```python
from build123d import *

# Parameters (mm, degrees)
SKETCH_1_W           = 512
SKETCH_1_H           = 80
EXTRUDE_1_DEPTH      = 6
SKETCH_2_R           = 2.55
CUT_EXTRUDE_1_DEPTH  = 7
EXTRUDE_2_DEPTH      = 6
SKETCH_3_R           = 2.1
SKETCH_3_W           = 7
SKETCH_3_H           = 6
CUT_EXTRUDE_11_DEPTH = 7
EXTRUDE_21_DEPTH     = 6
SKETCH_31_R          = 2.1
SKETCH_31_W          = 7
SKETCH_31_H          = 6
CUT_EXTRUDE_12_DEPTH = 7
EXTRUDE_22_DEPTH     = 6
SKETCH_32_R          = 2.1
SKETCH_32_W          = 7
SKETCH_32_H          = 6
CUT_EXTRUDE_13_DEPTH = 7
EXTRUDE_23_DEPTH     = 6
SKETCH_33_R          = 2.1
SKETCH_33_W          = 7
SKETCH_33_H          = 6
CUT_EXTRUDE_14_DEPTH = 7
SKETCH_35_R          = 2.1
SKETCH_35_W          = 7
SKETCH_35_H          = 6
CUT_EXTRUDE_16_DEPTH = 7
EXTRUDE_25_DEPTH     = 6
SKETCH_36_R          = 2.1
SKETCH_36_W          = 7
SKETCH_36_H          = 6
CUT_EXTRUDE_17_DEPTH = 7
SKETCH_37_R          = 2.1
SKETCH_37_W          = 7
SKETCH_37_H          = 6
CUT_EXTRUDE_18_DEPTH = 7


with BuildPart() as part:
    # Эскиз1 → Бобышка-Вытянуть1 (new body)
    with BuildSketch(Plane.XY):
        with Locations((256, -204.461538462)):
            Rectangle(SKETCH_1_W, SKETCH_1_H)
    extrude(amount=EXTRUDE_1_DEPTH)

    # Эскиз2 → Вырез-Вытянуть1 (cut, through all)
    with BuildSketch(Plane.XY.offset(6)):
        with Locations((376, -234.461538462)):
            Circle(SKETCH_2_R)
        with Locations((376, -214.461538462)):
            Circle(SKETCH_2_R)
        with Locations((136, -234.461538462)):
            Circle(SKETCH_2_R)
        with Locations((136, -214.461538462)):
            Circle(SKETCH_2_R)
    extrude(amount=-CUT_EXTRUDE_1_DEPTH, mode=Mode.SUBTRACT)

    # Эскиз21 → Бобышка-Вытянуть2 (add)
    with BuildSketch(Plane(origin=(462, -227.461538462, 0), x_dir=(0, -1, 0), z_dir=(0, 0, 1))):
        with BuildLine():
            Line((13, 53), (-13, 53))
            ThreePointArc((-13, 53), (-14.118033989, 52.736067977), (-15, 52))
            Line((-15, 52), (-16.2, 50.4))
            ThreePointArc((-16.2, 50.4), (-16.552786405, 50.105572809), (-17, 50))
            Line((-17, 50), (17, 50))
            ThreePointArc((17, 50), (16.552786405, 50.105572809), (16.2, 50.4))
            Line((16.2, 50.4), (15, 52))
            ThreePointArc((15, 52), (14.118033989, 52.736067977), (13, 53))
        make_face()
    extrude(amount=EXTRUDE_2_DEPTH)

    # Эскиз3 → Вырез-Вытянуть11 (cut, through all)
    with BuildSketch(Plane(origin=(462, -227.461538462, 6), x_dir=(0, -1, 0), z_dir=(0, 0, 1))):
        with Locations((0, 47)):
            Circle(SKETCH_3_R)
        with Locations((9.531849908, 47)):
            Rectangle(SKETCH_3_W, SKETCH_3_H)
        with Locations((-9.531849908, 47)):
            Rectangle(SKETCH_3_W, SKETCH_3_H)
    extrude(amount=-CUT_EXTRUDE_11_DEPTH, mode=Mode.SUBTRACT)

    # Эскиз22 → Бобышка-Вытянуть21 (add)
    with BuildSketch(Plane(origin=(462, -181.461538462, 0), x_dir=(0, -1, 0), z_dir=(0, 0, 1))):
        with BuildLine():
            Line((13, 53), (-13, 53))
            ThreePointArc((-13, 53), (-14.118033989, 52.736067977), (-15, 52))
            Line((-15, 52), (-16.2, 50.4))
            ThreePointArc((-16.2, 50.4), (-16.552786405, 50.105572809), (-17, 50))
            Line((-17, 50), (17, 50))
            ThreePointArc((17, 50), (16.552786405, 50.105572809), (16.2, 50.4))
            Line((16.2, 50.4), (15, 52))
            ThreePointArc((15, 52), (14.118033989, 52.736067977), (13, 53))
        make_face()
    extrude(amount=EXTRUDE_21_DEPTH)

    # Эскиз31 → Вырез-Вытянуть12 (cut, through all)
    with BuildSketch(Plane(origin=(462, -181.461538462, 6), x_dir=(0, -1, 0), z_dir=(0, 0, 1))):
        with Locations((0, 47)):
            Circle(SKETCH_31_R)
        with Locations((9.531849908, 47)):
            Rectangle(SKETCH_31_W, SKETCH_31_H)
        with Locations((-9.531849908, 47)):
            Rectangle(SKETCH_31_W, SKETCH_31_H)
    extrude(amount=-CUT_EXTRUDE_12_DEPTH, mode=Mode.SUBTRACT)

    # Эскиз23 → Бобышка-Вытянуть22 (add)
    with BuildSketch(Plane(origin=(50, -227.461538462, 0), x_dir=(0, 1, 0), z_dir=(0, 0, 1))):
        with BuildLine():
            Line((13, 53), (-13, 53))
            ThreePointArc((-13, 53), (-14.118033989, 52.736067977), (-15, 52))
            Line((-15, 52), (-16.2, 50.4))
            ThreePointArc((-16.2, 50.4), (-16.552786405, 50.105572809), (-17, 50))
            Line((-17, 50), (17, 50))
            ThreePointArc((17, 50), (16.552786405, 50.105572809), (16.2, 50.4))
            Line((16.2, 50.4), (15, 52))
            ThreePointArc((15, 52), (14.118033989, 52.736067977), (13, 53))
        make_face()
    extrude(amount=EXTRUDE_22_DEPTH)

    # Эскиз32 → Вырез-Вытянуть13 (cut, through all)
    with BuildSketch(Plane(origin=(50, -227.461538462, 6), x_dir=(0, 1, 0), z_dir=(0, 0, 1))):
        with Locations((0, 47)):
            Circle(SKETCH_32_R)
        with Locations((9.531849908, 47)):
            Rectangle(SKETCH_32_W, SKETCH_32_H)
        with Locations((-9.531849908, 47)):
            Rectangle(SKETCH_32_W, SKETCH_32_H)
    extrude(amount=-CUT_EXTRUDE_13_DEPTH, mode=Mode.SUBTRACT)

    # Эскиз24 → Бобышка-Вытянуть23 (add)
    with BuildSketch(Plane(origin=(50, -181.461538462, 0), x_dir=(0, 1, 0), z_dir=(0, 0, 1))):
        with BuildLine():
            Line((13, 53), (-13, 53))
            ThreePointArc((-13, 53), (-14.118033989, 52.736067977), (-15, 52))
            Line((-15, 52), (-16.2, 50.4))
            ThreePointArc((-16.2, 50.4), (-16.552786405, 50.105572809), (-17, 50))
            Line((-17, 50), (17, 50))
            ThreePointArc((17, 50), (16.552786405, 50.105572809), (16.2, 50.4))
            Line((16.2, 50.4), (15, 52))
            ThreePointArc((15, 52), (14.118033989, 52.736067977), (13, 53))
        make_face()
    extrude(amount=EXTRUDE_23_DEPTH)

    # Эскиз33 → Вырез-Вытянуть14 (cut, through all)
    with BuildSketch(Plane(origin=(50, -181.461538462, 6), x_dir=(0, 1, 0), z_dir=(0, 0, 1))):
        with Locations((0, 47)):
            Circle(SKETCH_33_R)
        with Locations((9.531849908, 47)):
            Rectangle(SKETCH_33_W, SKETCH_33_H)
        with Locations((-9.531849908, 47)):
            Rectangle(SKETCH_33_W, SKETCH_33_H)
    extrude(amount=-CUT_EXTRUDE_14_DEPTH, mode=Mode.SUBTRACT)

    # Эскиз35 → Вырез-Вытянуть16 (cut, through all)
    with BuildSketch(Plane(origin=(314, -214.461538462, 6), x_dir=(0, 1, 0), z_dir=(0, 0, 1))):
        with Locations((0, 47)):
            Circle(SKETCH_35_R)
        with Locations((9.531849908, 47)):
            Rectangle(SKETCH_35_W, SKETCH_35_H)
        with Locations((-9.531849908, 47)):
            Rectangle(SKETCH_35_W, SKETCH_35_H)
    extrude(amount=-CUT_EXTRUDE_16_DEPTH, mode=Mode.SUBTRACT)

    # Эскиз25 → Бобышка-Вытянуть25 (add)
    with BuildSketch(Plane(origin=(293, -194.461538462, 0), x_dir=(-1, 0, 0), z_dir=(0, 0, 1))):
        with BuildLine():
            Line((13, 53), (-13, 53))
            ThreePointArc((-13, 53), (-14.118033989, 52.736067977), (-15, 52))
            Line((-15, 52), (-16.2, 50.4))
            ThreePointArc((-16.2, 50.4), (-16.552786405, 50.105572809), (-17, 50))
            Line((-17, 50), (17, 50))
            ThreePointArc((17, 50), (16.552786405, 50.105572809), (16.2, 50.4))
            Line((16.2, 50.4), (15, 52))
            ThreePointArc((15, 52), (14.118033989, 52.736067977), (13, 53))
        make_face()
    extrude(amount=EXTRUDE_25_DEPTH)

    # Эскиз36 → Вырез-Вытянуть17 (cut, through all)
    with BuildSketch(Plane(origin=(293, -194.461538462, 6), x_dir=(-1, 0, 0), z_dir=(0, 0, 1))):
        with Locations((0, 47)):
            Circle(SKETCH_36_R)
        with Locations((9.531849908, 47)):
            Rectangle(SKETCH_36_W, SKETCH_36_H)
        with Locations((-9.531849908, 47)):
            Rectangle(SKETCH_36_W, SKETCH_36_H)
    extrude(amount=-CUT_EXTRUDE_17_DEPTH, mode=Mode.SUBTRACT)

    # Эскиз37 → Вырез-Вытянуть18 (cut, through all)
    with BuildSketch(Plane(origin=(293, -234.461538462, 6), x_dir=(1, 0, 0), z_dir=(0, 0, 1))):
        with Locations((0, 47)):
            Circle(SKETCH_37_R)
        with Locations((9.531849908, 47)):
            Rectangle(SKETCH_37_W, SKETCH_37_H)
        with Locations((-9.531849908, 47)):
            Rectangle(SKETCH_37_W, SKETCH_37_H)
    extrude(amount=-CUT_EXTRUDE_18_DEPTH, mode=Mode.SUBTRACT)


solid = part.part
```
Could you check a few things on this model? Use its own coordinates, in mm. Round coordinates to 2 decimals unless told otherwise and drop trailing zeros. Order: outer loops, then holes, each group sorted by start corner. A loop starts at its lowest first (then second) coordinate and runs counter-clockwise, first axis right, second up. Notation, with made-up numbers: M 44,15.25 L 91,15.25 A21 ccw 91,26.25 Z; hole C 79.5,3 d3. An arc over 180 degrees is marked long. One line per question, with ' | ' between items. Start each with the question number.
(1) For P1, Ø3, axis at x = 4, z = 2, coming from the -Y side; P2, Ø5, axis at x = 331.5, y = -195.5, coming from the -Z side; P3, Ø4, axis at x = 509, y = -227.46, coming from the -Z side, each with a flat end and sliding along its axis, tell me the tip position at first contact or that it passes through.
(2) Suppose I cut it at B-B on z = 1.95. Count the separate pieces of the cut face and the enclosed holes in it, then the cut area to 3 significant figures.
(3) Suppose I cut it at A-A on x = 389. List the corners of the cut face in (y, z) for me.
(4) Please list where these lines run through material, in increasing order: line 1 along Y through (x, z) = (376, 3.4); line 2 along Y through (x, z) = (293, 3.65); line 3 along X through (y, z) = (-214.5, 3.35).
Geometry results:
1) P1: y = -244.46 | P2: z = 0 | P3: through
2) separate pieces: 1 | enclosed holes: 25 | area: 40,700 mm²
3) outline: M -244.46,0 L -164.46,0 L -164.46,6 L -244.46,6 Z
4) line 1: -244.46 to -237.01, -231.91 to -217.01, -211.91 to -164.46 | line 2: -247.46 to -243.56, -239.36 to -189.56, -185.36 to -164.46 | line 3: -3 to 0, 6 to 133.45, 138.55 to 264.9, 269.1 to 373.45, 378.55 to 506, 512 to 515
